Geometry check sheet. Reference: drawing and pictorial views, mm from the part's lowest x, y, z. A direction names the side the tool comes from. Give positions to 0.01 mm unless a question says otherwise; leave off trailing zeros. Loops run counter-clockwise (first coordinate to the right, second up) from the corner with the lowest first, then second, coordinate; pieces in that order, holes last. Notation, with made-up numbers: (54, 33) -> (58, 33) arc R20 cw to (58, 52) -> close; hole circle Ø2 at (70, 29.25). An arc over 180 degrees is marked (long way). Write each question's results on one line, items separated by ' | '. Start each with the question number.
1. Cross-section at A-A on x = 2. Record the boundary of the cut face in (y, z) (1 decimal).
2. Mould release check, pull along Y, two halves, no side actions. Record for the marked faces 1, 2 and 3: +Y half, -Y half, draft (parallel to the pull), parting line (faces both ways), or undercut.
3. Material ranges on L1, parallel to Z at x = 2, y = 48 (1 decimal); L2, parallel to Y at x = 2, z = 30 (1 decimal); L3, parallel to Y at x = 5, z = 28 (1 decimal), recorded low to high. Write a range as from..to.
4. Gauge pin test, flat ends, axial feed: pin 1 Ø1.5 at (x, y) = (5.5, 28.5) entering from +Z; pin 2 Ø2 at (x, y) = (2.5, 38) entering from -Z (1 decimal). Record the tip position at first contact, or that the pin passes through.
5. Tool access check on the marked faces 4 and 5. Record the directions out of +Z, -Z, +X, -X, +Y, -Y that give a thin tool (end or side, any length) a straight path to the whole face; none if there is none.
6. Cross-section at D-D on y = 43.5. Record the boundary of the cut face in (x, z), and give its area (3 significant figures).
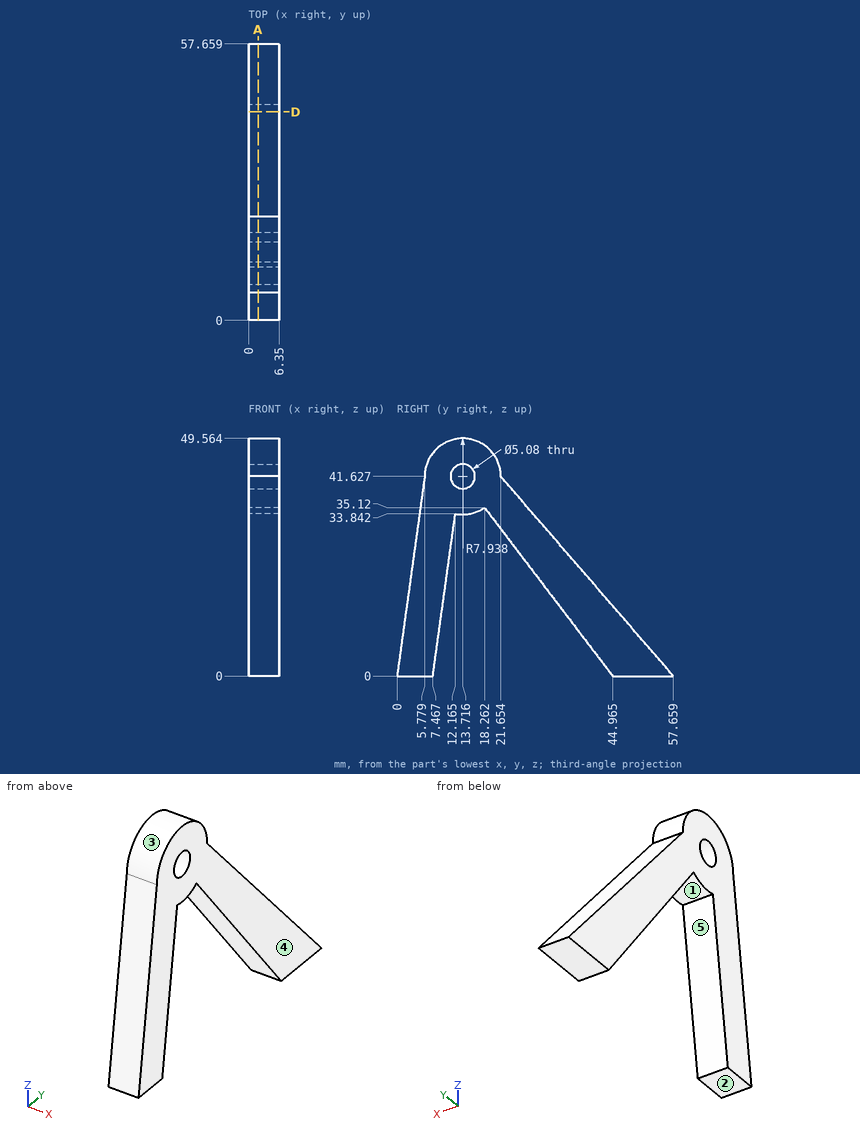
Geometry says:
1) outline: (0, 0) -> (7.5, 0) -> (12.2, 33.8) arc R7.9 ccw to (18.3, 35.1) -> (45, 0) -> (57.7, 0) -> (21.7, 41.6) arc R7.9 ccw to (5.8, 41.6) -> close; hole circle Ø5.1 at (13.7, 41.6)
2) face 1: undercut | face 2: draft | face 3: parting line
3) L1: 0..11.2 | L2: 4.2..11.6, 22.2..31.7 | L3: 3.9..11.4, 23.7..33.4
4) pin 1: z = 34.58 | pin 2: z = 7.8
5) face 4: +Z, -Z, +X, +Y, -Y | face 5: -Z, +X, -X
6) outline: (0, 1.93) -> (6.35, 1.93) -> (6.35, 16.37) -> (0, 16.37) -> close | area: 91.7 mm^2
